from build123d import *

# Parameters (mm, degrees)
SKETCH1_W           = 120
SKETCH1_H           = 120
BOSS_EXTRUDE2_DEPTH = 70
FILLET1_R           = 10
SHELL2_T            = -4
BOSS_EXTRUDE3_DEPTH = 30
CUT_EXTRUDE9_DEPTH  = 30


with BuildPart() as part:
    # Sketch1 → Boss-Extrude2 (new body)
    with BuildSketch(Plane.XY):
        Rectangle(SKETCH1_W, SKETCH1_H)
    extrude(amount=BOSS_EXTRUDE2_DEPTH)

    # Fillet1
    fillet1_edges = [part.edges().sort_by_distance(p)[0] for p in [
        (60, -60, 35),
        (-60, -60, 35),
        (-60, 60, 35),
        (60, 60, 35),
    ]]
    fillet(fillet1_edges, radius=FILLET1_R)

    # Shell2
    shell2_openings = [part.faces().sort_by_distance(p)[0] for p in [
        (0, 0, 70),
    ]]
    offset(amount=SHELL2_T, openings=shell2_openings, kind=Kind.INTERSECTION)

    # Sketch12 → Boss-Extrude3 (add)
    with BuildSketch(Plane.XY.offset(70)):
        with BuildLine():
            Line((-58, 50), (-58, -50))
            ThreePointArc((-58, -50), (-55.656854249, -55.656854249), (-50, -58))
            Line((-50, -58), (50, -58))
            ThreePointArc((50, -58), (55.656854249, -55.656854249), (58, -50))
            Line((58, -50), (58, 50))
            ThreePointArc((58, 50), (55.656854249, 55.656854249), (50, 58))
            Line((50, 58), (-50, 58))
            ThreePointArc((-50, 58), (-55.656854249, 55.656854249), (-58, 50))
        make_face()
    extrude(amount=BOSS_EXTRUDE3_DEPTH)

    # Sketch14 → Cut-Extrude9 (cut)
    with BuildSketch(Plane.XY.offset(100)):
        with BuildLine():
            Line((50, 56), (-50, 56))
            ThreePointArc((-50, 56), (-54.242640687, 54.242640687), (-56, 50))
            Line((-56, 50), (-56, -50))
            ThreePointArc((-56, -50), (-54.242640687, -54.242640687), (-50, -56))
            Line((-50, -56), (50, -56))
            ThreePointArc((50, -56), (54.242640687, -54.242640687), (56, -50))
            Line((56, -50), (56, 50))
            ThreePointArc((56, 50), (54.242640687, 54.242640687), (50, 56))
        make_face()
    extrude(amount=-CUT_EXTRUDE9_DEPTH, mode=Mode.SUBTRACT)


solid = part.part
CAD build for the part. Positions are in the model's coordinates, mm. A direction names the side the tool comes from. Round coordinates to 2 decimals unless told otherwise and drop trailing zeros. Loops run counter-clockwise (first coordinate to the right, second up) from the corner with the lowest first, then second, coordinate; pieces in that order, holes last.
(1) Which spindle directions (+Z, -Z, +X, -X, +Y, -Y) get a long thin tool onto all of the face, cutting with end or side? Do faces 4 (the cylindrical face through (-55.594, 55.719, 84.79)), 5 (the flat face through (58, -1, 85)), 6 (the cylindrical face through (55.594, -55.719, 84.79)). Say none if no direction does.
(2) Cut at D-D (z = 92). Give the cut face in (x, y).
(3) Two-plate mould, pull along X, no slides. Class faces 1 (the cylindrical face through (55.719, 55.594, 84.79)), 2 (the flat face through (-56, 1, 53)), 3 (the cylindrical face through (-55.719, -55.594, 84.79)): +X half, -X half, draft (parallel to the pull), parting line (faces both ways), or undercut.
(4) Cut at B-B (x = 20). Give the cut face in (y, z).
(5) Wall check: line 1 along X through (y, z) = (4, 4.5); line 2 along X through (y, z) = (-20.5, 79). Give the ranges that are in metal, low to high.
(6) Drop flat-ended pins along their axis: pin 1 (1 mm diameter, centred on y = -33, z = 75.5, fed in from -X); pin 2 (1.5 mm diameter, centred on x = 2.5, y = -20, fed in from -Z); pin 3 (1 mm diameter, centred on x = 20, y = 36.5, fed in from +Z); pin 4 (9 mm diameter, centred on x = 19, z = 88, fed in from -Y). Give the stop position or say it passes through.
(7) Cut at A-A (z = 21). Give the cut face in (x, y), plus the area to 3 significant figures.
Findings below:
1. face 4: +Z, -X, +Y
1. face 5: +Z, +X, +Y, -Y
1. face 6: +Z, +X, -Y
2. outline: (-58, -50) arc R8 ccw to (-50, -58) - (50, -58) arc R8 ccw to (58, -50) - (58, 50) arc R8 ccw to (50, 58) - (-50, 58) arc R8 ccw to (-58, 50) - close; hole (-56, -50) arc R6 ccw to (-50, -56) - (50, -56) arc R6 ccw to (56, -50) - (56, 50) arc R6 ccw to (50, 56) - (-50, 56) arc R6 ccw to (-56, 50) - close
3. face 1: +X half
3. face 2: undercut
3. face 3: -X half
4. outline: (-60, 0) - (60, 0) - (60, 70) - (58, 70) - (58, 100) - (56, 100) - (56, 4) - (-56, 4) - (-56, 100) - (-58, 100) - (-58, 70) - (-60, 70) - close
5. line 1: x = -60 to -56, 56 to 60
5. line 2: x = -58 to -56, 56 to 58
6. pin 1: stops at x = -58
6. pin 2: stops at z = 0
6. pin 3: stops at z = 4
6. pin 4: stops at y = -58
7. outline: (-60, -50) arc R10 ccw to (-50, -60) - (50, -60) arc R10 ccw to (60, -50) - (60, 50) arc R10 ccw to (50, 60) - (-50, 60) arc R10 ccw to (-60, 50) - close; hole (-56, -50) arc R6 ccw to (-50, -56) - (50, -56) arc R6 ccw to (56, -50) - (56, 50) arc R6 ccw to (50, 56) - (-50, 56) arc R6 ccw to (-56, 50) - close
7. area: 1,800 mm2
